Work out the finished part from the listing and answer in its coordinate system (mm). A direction names the side the tool comes from. Round coordinates to 2 decimals unless told otherwise and drop trailing zeros. Order: outer loops, then holes, each group sorted by start corner. A loop starts at its lowest first (then second) coordinate and runs counter-clockwise, first axis right, second up.
from build123d import *

# Parameters (mm, degrees)
PAD033_DEPTH            = 28.5
POCKET033_DEPTH         = 80
PAD034_DEPTH            = 44
POCKET034_DEPTH         = 80
POCKET035_DEPTH         = 65
POCKET035_DEPTH_BACK    = 100
SKETCH079_R             = 8.25
POCKET036_DEPTH         = 15
SKETCH080_R             = 8.25
POCKET037_DEPTH         = 19
POCKET038_DEPTH         = 14
POCKET039_DEPTH         = 12
SKETCH083_R             = 7.5
SKETCH083_R_2           = 2.75
POCKET040_DEPTH         = 50
SKETCH103_R             = 3.2
POCKET059_DEPTH         = 2
POCKET059_DEPTH_BACK    = 100
POCKET060_DEPTH         = 40
FILLET001_R             = 1
BODY016_PLACEMENT_ANGLE = 204.436


with BuildPart() as part:
    # Sketch074 → Pad033 (new body)
    with BuildSketch(Plane.XY.offset(44.25)):
        with BuildLine():
            Line((25, 4), (89, 4))
            ThreePointArc((89, 4), (93.9497474683, 6.0502525317), (96, 11))
            Line((96, 11), (96, 55))
            ThreePointArc((96, 55), (93.9497474683, 59.9497474683), (89, 62))
            Line((89, 62), (25, 62))
            ThreePointArc((25, 62), (20.0502525317, 59.9497474683), (18, 55))
            Line((18, 55), (18, 11))
            ThreePointArc((18, 11), (20.0502525317, 6.0502525317), (25, 4))
        make_face()
    extrude(amount=-PAD033_DEPTH)

    # Sketch075 (on Face7 of Pad033) → Pocket033 (cut)
    with BuildSketch(Plane(origin=(18, 0, 0), x_dir=(0, -1, 0), z_dir=(-1, 0, 0))):
        Polygon((-62, 15.75), (-4, 42.1136915968), (-4, 15.75), align=None)
        Polygon((-62, 17.8863084032), (-4, 44.25), (-62, 44.25), align=None)
    extrude(amount=-POCKET033_DEPTH, mode=Mode.SUBTRACT)

    # Sketch076 → Pad034 (join)
    with BuildSketch(Plane.XY):
        with BuildLine():
            ThreePointArc((20.5, 11), (21.8180194847, 7.8180194847), (25, 6.5))
            Line((25, 6.5), (89, 6.5))
            ThreePointArc((89, 6.5), (92.1819805153, 7.8180194847), (93.5, 11))
            Line((93.5, 11), (93.5, 55))
            ThreePointArc((93.5, 55), (92.1819805153, 58.1819805153), (89, 59.5))
            Line((25, 59.5), (89, 59.5))
            ThreePointArc((25, 59.5), (21.8180194847, 58.1819805153), (20.5, 55))
            Line((20.5, 55), (20.5, 11))
        make_face()
    extrude(amount=PAD034_DEPTH)

    # Sketch077 (on Face22 of Pad034) → Pocket034 (cut)
    with BuildSketch(Plane.YZ.offset(93.5)):
        Polygon((6.5, 43.1136339829), (59.5, 19.0226744203), (59.5, 44), (6.5, 44), align=None)
    extrude(amount=-POCKET034_DEPTH, mode=Mode.SUBTRACT)

    # Sketch078 (on DatumPlane) → Pocket035 (cut, two sides)
    with BuildSketch(Plane(origin=(96, 11, 38.9318667489), x_dir=(1, 0, 0), z_dir=(0, -0.9103661509, 0.4138036628))) as pocket035_sk:
        Polygon((-75.5, -10.4307806183), (-51.5, -4), (-26.5, -4), (-2.5, -10.4307806183), (-2.5, -38), (-75.5, -38), align=None)
    extrude(amount=-POCKET035_DEPTH, mode=Mode.SUBTRACT)
    extrude(pocket035_sk.sketch, amount=POCKET035_DEPTH_BACK, mode=Mode.SUBTRACT)

    # Sketch079 (on Face23 of Pocket035) → Pocket036 (cut)
    with BuildSketch(Plane(origin=(-6.0175887265, 9.2931806721, 20.4449546454), x_dir=(0.9659258263, 0.1071002689, 0.2356200979), z_dir=(0.2588190451, -0.3997036449, -0.8793461765))):
        with Locations((39.8763421354, -8.3497089553)):
            Circle(SKETCH079_R)
        with Locations((39.8763421354, -34.3497089553)):
            Circle(SKETCH079_R)
    extrude(amount=-POCKET036_DEPTH, mode=Mode.SUBTRACT)

    # Sketch080 (on Face27 of Pocket036) → Pocket037 (cut)
    with BuildSketch(Plane(origin=(13.6541407108, 21.0865850616, 46.3903899454), x_dir=(0.9659258263, -0.1071002689, -0.2356200979), z_dir=(-0.2588190451, -0.3997036449, -0.8793461765))):
        with Locations((70.2392020615, -8.3497089553)):
            Circle(SKETCH080_R)
        with Locations((70.2392020615, -34.3497089553)):
            Circle(SKETCH080_R)
    extrude(amount=-POCKET037_DEPTH, mode=Mode.SUBTRACT)

    # Sketch081 (on Face27 of Pocket037) → Pocket038 (cut)
    with BuildSketch(Plane(origin=(-8.0881410873, 12.4908098313, 27.4797240575), x_dir=(0.9659258263, 0.1071002689, 0.2356200979), z_dir=(0.2588190451, -0.3997036449, -0.8793461765))):
        with BuildLine():
            ThreePointArc((30.25, -25.25), (32.5, -27.5), (34.75, -25.25))
            Line((34.75, -25.25), (34.75, -17.25))
            ThreePointArc((34.75, -17.25), (32.5, -15), (30.25, -17.25))
            Line((30.25, -25.25), (30.25, -17.25))
        make_face()
    extrude(amount=-POCKET038_DEPTH, mode=Mode.SUBTRACT)

    # Sketch082 (on Face33 of Pocket038) → Pocket039 (cut)
    with BuildSketch(Plane(origin=(15.7246930716, 24.2842142208, 53.4251593575), x_dir=(0.9659258263, -0.1071002689, -0.2356200979), z_dir=(-0.2588190451, -0.3997036449, -0.8793461765))):
        with BuildLine():
            ThreePointArc((75.25, -25.25), (77.5, -27.5), (79.75, -25.25))
            Line((79.75, -25.25), (79.75, -17.25))
            ThreePointArc((79.75, -17.25), (77.5, -15), (75.25, -17.25))
            Line((75.25, -25.25), (75.25, -17.25))
        make_face()
    extrude(amount=-POCKET039_DEPTH, mode=Mode.SUBTRACT)

    # Sketch083 → Pocket040 (cut)
    with BuildSketch(Plane.XY):
        with Locations((57, 33)):
            Circle(SKETCH083_R)
        with Locations((48, 48.5884572681)):
            Circle(SKETCH083_R_2)
        with Locations((66, 48.5884572681)):
            Circle(SKETCH083_R_2)
        with Locations((75, 33)):
            Circle(SKETCH083_R_2)
        with Locations((39, 33)):
            Circle(SKETCH083_R_2)
        with Locations((48, 17.4115427319)):
            Circle(SKETCH083_R_2)
        with Locations((66, 17.4115427319)):
            Circle(SKETCH083_R_2)
    extrude(amount=POCKET040_DEPTH, mode=Mode.SUBTRACT)

    # Sketch103 → Pocket059 (cut, two sides)
    with BuildSketch(Plane.XY.offset(32)) as pocket059_sk:
        with Locations((39, 33)):
            Circle(SKETCH103_R)
        with Locations((75, 33)):
            Circle(SKETCH103_R)
    extrude(amount=-POCKET059_DEPTH, mode=Mode.SUBTRACT)
    extrude(pocket059_sk.sketch, amount=POCKET059_DEPTH_BACK, mode=Mode.SUBTRACT)

    # Sketch142 → Pocket060 (cut)
    with BuildSketch(Plane.XY.offset(40)):
        with BuildLine():
            Line((18, 17.4), (20, 17.4))
            ThreePointArc((20, 17.4), (20.3535533906, 17.5464466094), (20.5, 17.9))
            Line((20.5, 17.9), (20.5, 26.9))
            ThreePointArc((20.5, 26.9), (20.3535533906, 27.2535533906), (20, 27.4))
            Line((20, 27.4), (18, 27.4))
            Line((18, 27.4), (18, 17.4))
        make_face()
        with BuildLine():
            Line((18, 43), (20, 43))
            ThreePointArc((20, 43), (20.3535533906, 43.1464466094), (20.5, 43.5))
            Line((20.5, 43.5), (20.5, 52.5))
            ThreePointArc((20.5, 52.5), (20.3535533906, 52.8535533906), (20, 53))
            Line((20, 53), (18, 53))
            Line((18, 53), (18, 43))
        make_face()
        with BuildLine():
            Line((96, 53), (94, 53))
            ThreePointArc((94, 53), (93.6464466094, 52.8535533906), (93.5, 52.5))
            Line((93.5, 52.5), (93.5, 43.5))
            ThreePointArc((93.5, 43.5), (93.6464466094, 43.1464466094), (94, 43))
            Line((94, 43), (96, 43))
            Line((96, 43), (96, 53))
        make_face()
        with BuildLine():
            Line((96, 17.4), (94, 17.4))
            ThreePointArc((93.5, 17.9), (93.6464466094, 17.5464466094), (94, 17.4))
            Line((93.5, 17.9), (93.5, 26.9))
            ThreePointArc((94, 27.4), (93.6464466094, 27.2535533906), (93.5, 26.9))
            Line((94, 27.4), (96, 27.4))
            Line((96, 27.4), (96, 17.4))
        make_face()
    extrude(amount=-POCKET060_DEPTH, mode=Mode.SUBTRACT)

    # Fillet001
    fillet001_edges = [part.edges().sort_by_distance(p)[0] for p in [
        (18, 53, 20.909072),
        (18, 43, 25.454536),
        (18, 27.4, 32.54546),
        (18, 17.4, 37.090924),
        (96, 53, 20.909072),
        (96, 43, 25.454536),
        (96, 27.4, 32.54546),
        (96, 17.4, 37.090924),
    ]]
    fillet(fillet001_edges, radius=FILLET001_R)


with BuildPart() as part_1:
    # Body016 placement: moved
    add(part.part.rotate(Axis((0, 0, 0), (1, 0, 0)), BODY016_PLACEMENT_ANGLE))


solid = part_1.part
Item 1: Given pin 1 (3.5 mm diameter, centred on y = -13.5, z = -38, fed in from -X); pin 2 (0.8 mm diameter, centred on x = 95, y = -18, fed in from +Z); pin 3 (6 mm diameter, centred on x = 34.5, y = -14.5, fed in from -Z), each flat-ended and moving along its own axis, determine where each tip first touches the part or whether it passes through.
Item 2: Find section B-B (x = 29.5). State how many separate pieces and enclosed holes the cut face has, plus the area to 3 significant figures.
Item 3: Find the intervals of material crossed by line 1 along Y through (x, z) = (39, -35.25); line 2 along X through (y, z) = (-6.5, -37.25); line 3 along Y through (x, z) = (89.5, -38), in increasing order.
Item 4: Find section A-A (x = 43.5). Write down the section's boundary in (y, z).
Item 5: A tool of negligible diameter and unlimited length cuts with its end or side. For faces 4 (the face through (56.55, 9.84, -37.37)), 5 (the face through (95.715, -0.137, -41.032)), 6 (the face through (18.285, -39.978, -40.862)), 7 (the face through (93.895, 12.006, -40.918)), 8 (the face through (22.855, -27.505, -40.079)), from which of +Z, -Z, +X, -X, +Y, -Y can it reach the whole face along a straight path? Write none if from no direction.
Item 6: For a pull along Y with two mould halves and no side action, classify faces 1 (the face through (57.448, -49.483, -40.973)), 2 (the face through (18, 4, -41)), 3 (the face through (63.97, -37.38, -39.67)) as released by +Y, released by -Y, zero draft, split by the parting line, or undercut.
Model answer:
1. pin 1: stops at x = 20.5
1. pin 2: stops at z = -39.99
1. pin 3: stops at z = -41.94
2. separate pieces: 3
2. enclosed holes: 0
2. area: 271 mm2
3. line 1: y = -49.34 to -38.85, -29.86 to -23.25, -17.21 to -12.85, -3.86 to 8.88
3. line 2: x = 20.5 to 22.98, 39.62 to 74.38, 91.02 to 93.5
3. line 3: y = -48.06 to -39.59, -29.12 to -13.59, -3.12 to 10.1
4. outline: (-49.93, -39.99) - (-49.05, -41.93) - (14.66, -41.94) - (13.78, -40) - (11.03, -40) - (9.09, -35.73) - (-49.12, -35.72) - (-47.18, -39.99) - close
5. face 4: +Z, +X, -X, +Y
5. face 5: -Z, +X
5. face 6: +Z, -X
5. face 7: +Z, +X, +Y
5. face 8: none
6. face 1: released by -Y
6. face 2: zero draft
6. face 3: undercut
